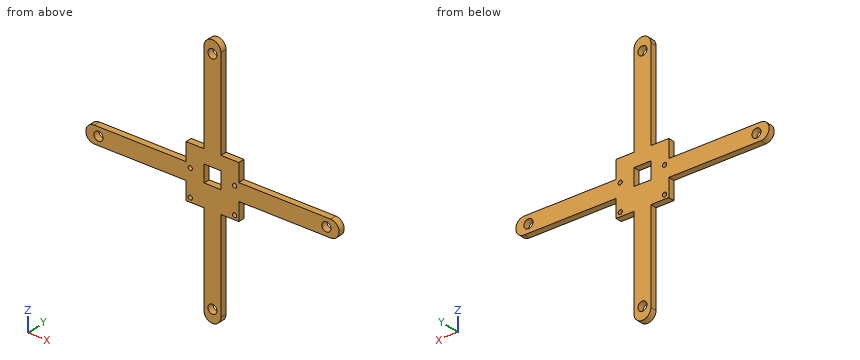
from build123d import *

# Parameters (mm, degrees)
SCHIZZO1_R                   = 1
SCHIZZO1_R_2                 = 2.15
SCHIZZO1_W                   = 8
SCHIZZO1_H                   = 8
ESTRUSIONE_ESTRUSIONE1_DEPTH = 3


with BuildPart() as part:
    # Schizzo1 → Estrusione-Estrusione1 (new body)
    with BuildSketch(Plane(origin=(0, 0, 0), x_dir=(1, 0, 0), z_dir=(0, 1, 0))):
        with BuildLine():
            Line((4, 55.99875276), (4, 12.5))
            Line((4, 12.5), (12.5, 12.5))
            Line((12.5, 12.5), (12.5, 4))
            Line((12.5, 4), (55.99875276, 4))
            ThreePointArc((55.99875276, 4), (60, 0), (55.99875276, -4))
            Line((55.99875276, -4), (12.5, -4))
            Line((12.5, -4), (12.5, -12.5))
            Line((12.5, -12.5), (4, -12.5))
            Line((4, -12.5), (4, -55.99875276))
            ThreePointArc((4, -55.99875276), (0, -59.99875276), (-4, -55.99875276))
            Line((-4, -55.99875276), (-4, -12.5))
            Line((-4, -12.5), (-12.5, -12.5))
            Line((-12.5, -12.5), (-12.5, -4))
            Line((-12.5, -4), (-55.99875276, -4))
            ThreePointArc((-55.99875276, -4), (-60.000000389, 0), (-55.99875276, 4))
            Line((-55.99875276, 4), (-12.5, 4))
            Line((-12.5, 4), (-12.5, 12.5))
            Line((-12.5, 12.5), (-4, 12.5))
            Line((-4, 12.5), (-4, 55.99875276))
            ThreePointArc((-4, 55.99875276), (0, 60), (4, 55.99875276))
        make_face()
        with Locations(Location((-10.5, 10.5, 0), (0, 0, 270))):
            Circle(SCHIZZO1_R, mode=Mode.SUBTRACT)
        with Locations(Location((10.5, 10.5, 0), (0, 0, 270))):
            Circle(SCHIZZO1_R, mode=Mode.SUBTRACT)
        with Locations(Location((-10.5, -2, 0), (0, 0, 270))):
            Circle(SCHIZZO1_R, mode=Mode.SUBTRACT)
        with Locations(Location((10.5, -2, 0), (0, 0, 270))):
            Circle(SCHIZZO1_R, mode=Mode.SUBTRACT)
        with Locations(Location((-54, 0, 0), (0, 0, 270))):
            Circle(SCHIZZO1_R_2, mode=Mode.SUBTRACT)
        with Locations(Location((0, 54, 0), (0, 0, 270))):
            Circle(SCHIZZO1_R_2, mode=Mode.SUBTRACT)
        with Locations(Location((54, 0, 0), (0, 0, 270))):
            Circle(SCHIZZO1_R_2, mode=Mode.SUBTRACT)
        with Locations(Location((0, -54, 0), (0, 0, 270))):
            Circle(SCHIZZO1_R_2, mode=Mode.SUBTRACT)
        with Locations((0, -2)):
            Rectangle(SCHIZZO1_W, SCHIZZO1_H, mode=Mode.SUBTRACT)
    extrude(amount=ESTRUSIONE_ESTRUSIONE1_DEPTH)


solid = part.part
Read the model definition and answer for the solid it produces. Units are mm, in the model's axes. Round coordinates to 2 decimals unless told otherwise and drop trailing zeros. Write each loop counter-clockwise with the first axis right and the second up, starting at its lowest first coordinate (ties: lowest second). Pieces come first, ordered by that corner, then holes.
1. The part is cut by section A-A, the plane x = -54. Determine the outline of the cut face in (y, z), then the cut area to 3 significant figures.
2. Given pin 1 Ø1.5 at (y, z) = (1.5, 8) entering from +X; pin 2 Ø0.9 at (x, y) = (1, 2) entering from -Z; pin 3 Ø0.9 at (y, z) = (1, 41.5) entering from +X, each flat-ended and moving along its own axis, determine where each tip first touches the part or whether it passes through.
3. The part is cut by section D-D, the plane y = 0.7. State how many separate pieces and enclosed holes the cut face has, then the cut area to 3 significant figures.
4. The part is cut by section B-B, the plane z = -54. Determine the outline of the cut face in (x, y), then the cut area to 3 significant figures.
5. The part is cut by section C-C, the plane x = 0. Determine the outline of the cut face in (y, z), then the cut area to 3 significant figures.
6. Straight lines are drawn through the part: L1, parallel to X at y = 1.95, z = -54; L2, parallel to Z at x = -1, y = 1.85; L3, parallel to X at y = 1.3, z = 22. For each, find the intervals that lie inside material, in ascending order.
Values:
1. outline: (0, -4) - (3, -4) - (3, -2.15) - (0, -2.15) - close; (0, 2.15) - (3, 2.15) - (3, 4) - (0, 4) - close
1. area: 11.1 mm2
2. pin 1: stops at x = 12.5
2. pin 2: stops at z = -59.96
2. pin 3: stops at x = 4
3. separate pieces: 1
3. enclosed holes: 9
3. area: 1,980 mm2
4. outline: (-4, 0) - (-2.15, 0) - (-2.15, 3) - (-4, 3) - close; (2.15, 0) - (4, 0) - (4, 3) - (2.15, 3) - close
4. area: 11.1 mm2
5. outline: (0, -60) - (3, -60) - (3, -56.15) - (0, -56.15) - close; (0, -51.85) - (3, -51.85) - (3, -2) - (0, -2) - close; (0, 6) - (3, 6) - (3, 51.85) - (0, 51.85) - close; (0, 56.15) - (3, 56.15) - (3, 60) - (0, 60) - close
5. area: 310 mm2
6. L1: x = -4 to -2.15, 2.15 to 4
6. L2: z = -59.87 to -55.9, -52.1 to -2, 6 to 52.1, 55.9 to 59.87
6. L3: x = -4 to 4
